Could you check a few things on this drawing? It's one solid part, dimensions in mm from its lowest x, y, z. A direction names the side the tool comes from. Give positions to 0.01 mm unless a question says otherwise; leave off trailing zeros. Loops run counter-clockwise (first coordinate to the right, second up) from the corner with the lowest first, then second, coordinate; pieces in that order, holes last. Notation, with made-up numbers: M 28.5,85 L 37.5,85 A18 cw 37.5,107 Z; hole C 75.5,-13 d10. An arc over 180 degrees is marked long. Return JSON: item names as keys, results as strings. Group by question number.
1. If we section it at B-B (z = 33): Write out the boundary of the cut face in (x, y) (1 decimal).
2. For the marked faces 1 and 2, which set-ups out of +Z, -Z, +X, -X, +Y, -Y let a thin tool reach every point of the face, with its end or its side?
3. If we section it at A-A (x = 9.5): Write out the boundary of the cut face in (y, z).
4. Please list where these lines run through material, in increasing order: line 1 (X direction, y = 50, z = 46); line 2 (Z direction, x = 68, y = 43) (1 decimal); line 3 (Z direction, x = 6, y = 51.5).
5. If we section it at D-D (z = 54): Write out the boundary of the cut face in (x, y), plus the area to 3 significant figures.
6. If we section it at C-C (y = 26): Write out the boundary of the cut face in (x, z).
7. For pin 1 (4 mm diameter, centred on x = 39.5, z = 50.5, fed in from +Y); pin 2 (8 mm diameter, centred on x = 64, y = 71.5, fed in from -Z); pin 3 (10 mm diameter, centred on x = 58.5, y = 15.5, fed in from +Z); pin 4 (10 mm diameter, centred on x = 54, z = 25.5, fed in from +Y), each with a flat end and sliding along its axis, tell me the tip position at first contact or that it passes through.
8. If we mould it in two halves opening along Z, with no side actions, what happens to the marked faces 3, 4 and 5? For each: +Z half, -Z half, draft (parallel to the pull), parting line (faces both ways), or undercut.
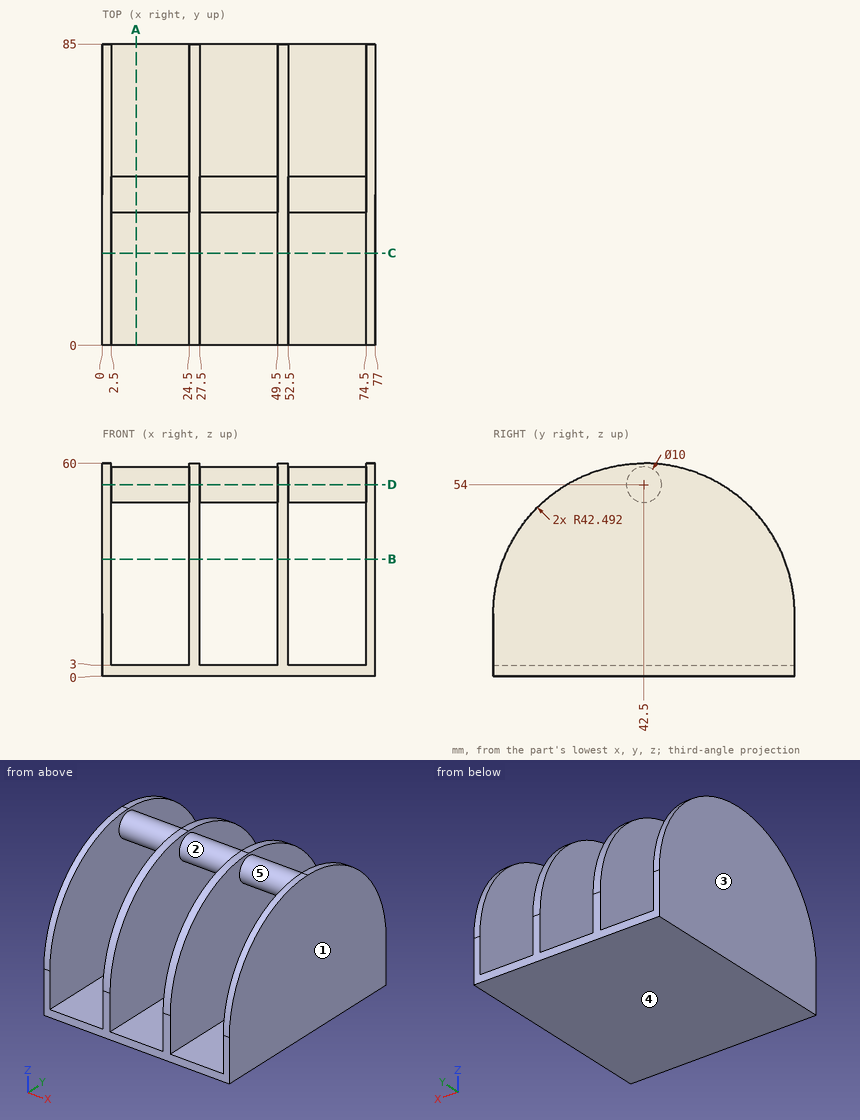
Answer:
{
 "1": {"outline": "M 0,2.9 L 2.5,2.9 L 2.5,82.1 L 0,82.1 Z; M 24.5,2.9 L 27.5,2.9 L 27.5,82.1 L 24.5,82.1 Z; M 49.5,2.9 L 52.5,2.9 L 52.5,82.1 L 49.5,82.1 Z; M 74.5,2.9 L 77,2.9 L 77,82.1 L 74.5,82.1 Z"},
 "2": {"face 1": "+Z, -Z, +X, +Y, -Y", "face 2": "none"},
 "3": {"outline": "M 0,0 L 85,0 L 85,3 L 0,3 Z; C 42.5,54 d10"},
 "4": {"line 1": "x = 0 to 2.5, 24.5 to 27.5, 49.5 to 52.5, 74.5 to 77", "line 2": "z = 0 to 3, 49 to 59", "line 3": "z = 0 to 3"},
 "5": {"outline": "M 0,20.72 L 2.5,20.72 L 2.5,37.5 L 24.5,37.5 L 24.5,20.72 L 27.5,20.72 L 27.5,37.5 L 49.5,37.5 L 49.5,20.72 L 52.5,20.72 L 52.5,37.5 L 74.5,37.5 L 74.5,20.72 L 77,20.72 L 77,64.28 L 74.5,64.28 L 74.5,47.5 L 52.5,47.5 L 52.5,64.28 L 49.5,64.28 L 49.5,47.5 L 27.5,47.5 L 27.5,64.28 L 24.5,64.28 L 24.5,47.5 L 2.5,47.5 L 2.5,64.28 L 0,64.28 Z", "area": "1,140 mm²"},
 "6": {"outline": "M 0,0 L 77,0 L 77,56.67 L 74.5,56.67 L 74.5,3 L 52.5,3 L 52.5,56.67 L 49.5,56.67 L 49.5,3 L 27.5,3 L 27.5,56.67 L 24.5,56.67 L 24.5,3 L 2.5,3 L 2.5,56.67 L 0,56.67 Z"},
 "7": {"pin 1": "stops at y = 47.27", "pin 2": "stops at z = 0", "pin 3": "stops at z = 3", "pin 4": "stops at y = 84.88"},
 "8": {"face 3": "draft", "face 4": "-Z half", "face 5": "undercut"}
}
